Could you check a few things on this model? Use its own coordinates, in mm. Coordinates: 2 decimals unless noted, no trailing zeros. Loops run counter-clockwise (first coordinate to the right, second up) from the corner with the lowest first, then second, coordinate; pieces in that order, holes last. Notation, with made-up numbers: (55.25, 64) - (86.25, 64) arc R14 ccw to (86.25, 70) - close; hole circle Ø1 at (10.25, 20). An arc over 180 degrees is marked (long way). Use CSV: the item, a comma, the result in double quotes.
from build123d import *


with BuildPart() as f1:
    # F0 (on Top) → F1 (revolve)
    with BuildSketch(Plane.XY):
        with BuildLine():
            ThreePointArc((-27.5, -2.5), (-28.232233047, -0.732233047), (-30, 0))
            ThreePointArc((-30, 0), (-31.767766953, -0.732233047), (-32.5, -2.5))
            Line((-32.5, -2.5), (-33.6200716846, -5))
            Line((-33.6200716846, -5), (-28.6200716846, -5))
            Line((-28.6200716846, -5), (-27.5, -2.5))
        make_face()
        Polygon((-36.3799283154, -22.32), (-28.6200716846, -5), (-33.6200716846, -5), (-41.3799283154, -22.32), align=None)
        with BuildLine():
            Line((-37.5, -24.82), (-36.3799283154, -22.32))
            Line((-36.3799283154, -22.32), (-41.3799283154, -22.32))
            Line((-41.3799283154, -22.32), (-42.5, -24.82))
            ThreePointArc((-42.5, -24.82), (-41.767766953, -26.587766953), (-40, -27.32))
            ThreePointArc((-40, -27.32), (-38.232233047, -26.587766953), (-37.5, -24.82))
        make_face()
    revolve(axis=Axis((0, -13.66, 0), (0, -1, 0)))


solid = f1.part
(1) Please list where these lines run through material, in increasing order: line 1 (Z direction, x = -13.5, y = -9); line 2 (X direction, y = -12.25, z = -15); line 3 (Z direction, x = -22, y = -23.25).
Computed:
line 1,"z = -32.74 to -27.25, 27.25 to 32.74"
line 2,"x = -33.68 to -28.12, 28.12 to 33.68"
line 3,"z = -35.54 to -29.5, 29.5 to 35.54"
(2) Suppose I cut it at A-A (y = -19.25). Write out the boundary of the cut face in (x, z).
Computed:
outline,"circle Ø80.01 at (0, 0); hole circle Ø70.01 at (0, 0)"
(3) Will these pins go through, and if not, where does the flat tip stop? pin 1 (8 mm diameter, centred on x = -26, y = -3.5, fed in from -Z); pin 2 (4 mm diameter, centred on y = -11.5, z = 19.5, fed in from +X); pin 3 (2 mm diameter, centred on x = -22.5, y = -23, fed in from +Z).
Computed:
pin 1,"stops at z = -25.26"
pin 2,"stops at x = 32.47"
pin 3,"stops at z = 35.91"
